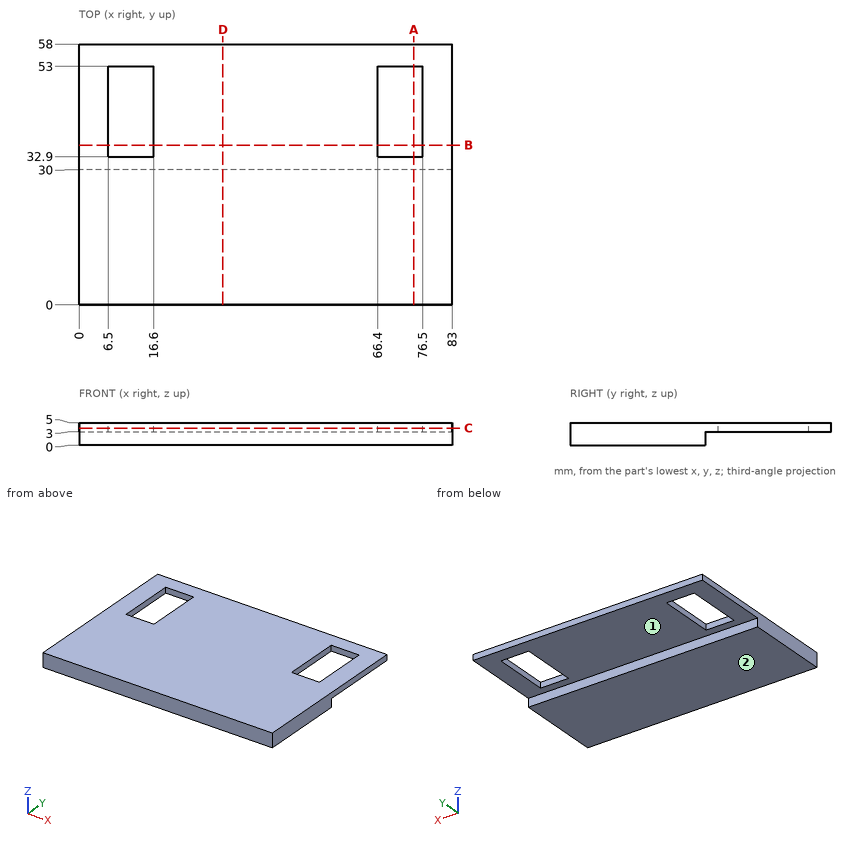
Geometry check sheet. Reference: drawing and pictorial views, mm from the part's lowest x, y, z. A direction names the side the tool comes from. Round coordinates to 2 decimals unless told otherwise and drop trailing zeros. Loops run counter-clockwise (first coordinate to the right, second up) from the corner with the lowest first, then second, coordinate; pieces in that order, holes last. Notation, with made-up numbers: (36.5, 25) - (62.5, 25) arc R19 cw to (62.5, 41) - close; hole circle Ø4 at (-28.75, 80). An arc over 180 degrees is marked (long way). Use a Markdown table: item, result. Add a question column.
1. Access from +Z, -Z, +X, -X, +Y, -Y to the whole of each face (thin tool, end or side, straight path). Record for the marked faces 1 and 2.
2. Thickness scan on probe 1 along X at (y, z) = (52, 3.9); probe 2 along Y at (x, z) = (14, 4.6); probe 3 along Y at (x, z) = (65.5, 2.95). Record the ranges inside material, lowest first. Write a range as [from, to].
3. Gauge pin test, flat ends, axial feed: pin 1 (2 mm diameter, centred on x = 9, y = 42.5, fed in from +Z); pin 2 (6 mm diameter, centred on x = 60.5, y = 52, fed in from -Z); pin 3 (1.5 mm diameter, centred on x = 33.5, z = 2, fed in from +Y). Record the tip position at first contact, or that the pin passes through.
4. Section check C-C, the plane z = 3.8. Record the boundary of the cut face in (x, y).
5. Section check A-A, the plane x = 74.5. Record the boundary of the cut face in (y, z), plus the area to 3 significant figures.
6. Section check B-B, the plane y = 35.5. Record the boundary of the cut face in (x, z).
7. Section check D-D, the plane x = 32. Record the boundary of the cut face in (y, z), plus the area to 3 significant figures.
Checks:
| question | item | result |
|---|---|---|
| 1 | face 1 | -Z, +X, -X, +Y |
| 1 | face 2 | -Z, +X, -X, +Y, -Y |
| 2 | probe 1 | x = [0, 6.5], [16.6, 66.4], [76.5, 83] |
| 2 | probe 2 | y = [0, 32.9], [53, 58] |
| 2 | probe 3 | y = [0, 30] |
| 3 | pin 1 | passes through |
| 3 | pin 2 | stops at z = 3 |
| 3 | pin 3 | stops at y = 30 |
| 4 | outline | (0, 0) - (83, 0) - (83, 58) - (0, 58) - close; hole (6.5, 32.9) - (16.6, 32.9) - (16.6, 53) - (6.5, 53) - close; hole (66.4, 32.9) - (76.5, 32.9) - (76.5, 53) - (66.4, 53) - close |
| 5 | outline | (0, 0) - (30, 0) - (30, 3) - (32.9, 3) - (32.9, 5) - (0, 5) - close; (53, 3) - (58, 3) - (58, 5) - (53, 5) - close |
| 5 | area | 166 mm^2 |
| 6 | outline | (0, 3) - (6.5, 3) - (6.5, 5) - (0, 5) - close; (16.6, 3) - (66.4, 3) - (66.4, 5) - (16.6, 5) - close; (76.5, 3) - (83, 3) - (83, 5) - (76.5, 5) - close |
| 7 | outline | (0, 0) - (30, 0) - (30, 3) - (58, 3) - (58, 5) - (0, 5) - close |
| 7 | area | 206 mm^2 |
